Work out the finished part from the listing and answer in its coordinate system (mm). A direction names the side the tool comes from. Give positions to 0.01 mm unless a question says otherwise; leave off trailing zeros. Order: outer loops, then holes, each group sorted by start corner. A loop starts at its lowest first (then second) coordinate and runs counter-clockwise, first axis right, second up. Notation, with made-up numbers: M 49,-29.5 L 74,-29.5 A15 cw 74,-13.5 Z; hole C 78,39 d11. An arc over 180 degrees is marked long. One line per item, written item: value.
from build123d import *

# Parameters (mm, degrees)
F1_DEPTH = 19.05
F3_DEPTH = 25
F4_R     = 50
F5_R     = 25
F6_R     = 50
F7_R     = 3.175
F8_DEPTH = 25
F9_R     = 100


with BuildPart() as f1:
    # F0 (on Front) → F1 (new body)
    with BuildSketch(Plane.XZ):
        Polygon((-750, 0), (0, 0), (0, 350), (-150, 350), (-300, 250), (-750, 175), align=None)
    extrude(amount=F1_DEPTH)

    # F2 (on face) → F3 (cut)
    with BuildSketch(Plane.XZ.offset(19.05)):
        Polygon((-325, 195.143646), (-700, 132.643646), (-700, 50), (-325, 50), align=None)
        Polygon((-134.861218, 300), (-275, 206.574145), (-275, 50), (-50, 50), (-50, 300), align=None)
    extrude(amount=-F3_DEPTH, mode=Mode.SUBTRACT)

    # F4
    f4_edges = [f1.edges().sort_by_distance(p)[0] for p in [
        (-325, -9.525, 195.143646),
        (-325, -9.525, 50),
        (-275, -9.525, 206.574145),
        (-134.861218, -9.525, 300),
        (-50, -9.525, 300),
        (-50, -9.525, 50),
        (-275, -9.525, 50),
    ]]
    fillet(f4_edges, radius=F4_R)

    # F5
    f5_edges = [f1.edges().sort_by_distance(p)[0] for p in [
        (-700, -9.525, 132.643646),
        (-700, -9.525, 50),
    ]]
    fillet(f5_edges, radius=F5_R)

    # F6
    f6_edges = [f1.edges().sort_by_distance(p)[0] for p in [
        (-750, -9.525, 175),
        (-750, -9.525, 0),
        (-150, -9.525, 350),
    ]]
    fillet(f6_edges, radius=F6_R)

    # F7 (on face) → F8 (cut)
    with BuildSketch(Plane.XZ.offset(19.05)):
        with Locations((-25, 275)):
            Circle(F7_R)
        with Locations((-25, 75)):
            Circle(F7_R)
    extrude(amount=-F8_DEPTH, mode=Mode.SUBTRACT)

    # F9
    f9_edges = [f1.edges().sort_by_distance(p)[0] for p in [
        (-300, -9.525, 250),
    ]]
    fillet(f9_edges, radius=F9_R)


solid = f1.part
(1) Determine the mould class of faces 3 (the flat face through (0, -9, 173)), 4 (the flat face through (-511.99, -9.39, 214.67)), 5 (the flat face through (-50, -10, 174)) for opening direction X: pulls with the +X half, pulls with the -X half, needs draft (parallel to the pull), parting line crosses it, or undercut.
Findings:
face 3: pulls with the +X half
face 4: pulls with the -X half
face 5: undercut
(2) Find the intervals of material crossed by probe 1 along X at (y, z) = (-2.25, 100.5); probe 2 along Z at (x, y) = (-25, -12.75) (3 decimals); probe 3 along X at (y, z) = (-11.5, 275) (3 decimals), in increasing order. Write a range as from..to.
Findings:
probe 1: x = -750..-700, -325..-275, -50..0
probe 2: z = 0..71.825, 78.175..271.825, 278.175..350
probe 3: x = -262.5..-172.361, -56.699..-28.175, -21.825..0
(3) Given P1, Ø1, axis at x = -335.5, y = -14, coming from the +Z side; P2, Ø9.5, axis at x = -543.5, y = -10.5, coming from the +Z side; P3, Ø6, axis at x = -570, y = -16.5, coming from the +Z side, each flat-ended and moving along its own axis, determine where each tip first touches the part or whether it passes through.
Findings:
P1: stops at z = 244.17
P2: stops at z = 210.21
P3: stops at z = 205.5
(4) Section A-A, the plane y = -5.75 is taken. Give the number of separate pieces and of enclosed holes in the cut face, then the cut area to 3 significant figures.
Findings:
separate pieces: 1
enclosed holes: 4
area: 103,000 mm^2
(5) Which of the six approach directions +Z, -Z, +X, -X, +Y, -Y give full straight-line access (tool end or side, diameter ignored) to faces 1 (the flat face through (-199.36, -9.66, 257)), 2 (the cylindrical face through (-734.964, -9.658, 14.258))?
Findings:
face 1: +Y, -Y
face 2: -Z, -X, +Y, -Y
(6) Section C-C, the plane z = 323 is taken. Give the vertices of the cut face in (x, y).
Findings:
outline: M -190.5,-19.05 L 0,-19.05 L 0,0 L -190.5,0 Z
(7) Section B-B, the plane x = -645 is taken. Give the vertices of the cut face in (y, z), then the cut area to 3 significant figures.
Findings:
outline: M -19.05,0 L 0,0 L 0,50 L -19.05,50 Z; M -19.05,141.81 L 0,141.81 L 0,192.5 L -19.05,192.5 Z
area: 1,920 mm^2
